from build123d import *

# Parameters (mm, degrees)
SKETCH1_R           = 3
BOSS_EXTRUDE3_DEPTH = 8
SKETCH2_R           = 4.75
CUT_EXTRUDE1_DEPTH  = 109.271164213


with BuildPart() as part:
    # Sketch1 → Boss-Extrude3 (new body)
    # profile 1 of 5: a face of its own
    with BuildSketch(Plane.XY):
        with BuildLine():
            ThreePointArc((76.35, 0), (53.987602744, 53.987602744), (0, 76.35))
            ThreePointArc((0, 76.35), (-62.014972319, 44.536116897), (-72.348554199, -24.392810524))
            ThreePointArc((-72.348554199, -24.392810524), (-44.536116897, -62.014972319), (0, -76.35))
            ThreePointArc((0, -76.35), (53.987602744, -53.987602744), (76.35, 0))
        make_face()
        Polygon((-27.25, -54.236860279), (-24.5, -59), (-27.25, -63.763139721), (-32.75, -63.763139721), (-35.5, -59), (-32.75, -54.236860279), align=None, mode=Mode.SUBTRACT)
        Polygon((54.236860279, -27.25), (59, -24.5), (63.763139721, -27.25), (63.763139721, -32.75), (59, -35.5), (54.236860279, -32.75), align=None, mode=Mode.SUBTRACT)
        Polygon((-54.236860279, 27.25), (-59, 24.5), (-63.763139721, 27.25), (-63.763139721, 32.75), (-59, 35.5), (-54.236860279, 32.75), align=None, mode=Mode.SUBTRACT)
        Polygon((27.25, 54.236860279), (24.5, 59), (27.25, 63.763139721), (32.75, 63.763139721), (35.5, 59), (32.75, 54.236860279), align=None, mode=Mode.SUBTRACT)
    # profile 2 of 5: a face of its own
    with BuildSketch(Plane.XY):
        Polygon((-63.763139721, 32.75), (-63.763139721, 27.25), (-59, 24.5), (-54.236860279, 27.25), (-54.236860279, 32.75), (-59, 35.5), align=None)
        with Locations((-59, 30)):
            Circle(SKETCH1_R, mode=Mode.SUBTRACT)
    # profile 3 of 5: a face of its own
    with BuildSketch(Plane.XY):
        Polygon((32.75, 63.763139721), (27.25, 63.763139721), (24.5, 59), (27.25, 54.236860279), (32.75, 54.236860279), (35.5, 59), align=None)
        with Locations((30, 59)):
            Circle(SKETCH1_R, mode=Mode.SUBTRACT)
    # profile 4 of 5: a face of its own
    with BuildSketch(Plane.XY):
        Polygon((63.763139721, -32.75), (63.763139721, -27.25), (59, -24.5), (54.236860279, -27.25), (54.236860279, -32.75), (59, -35.5), align=None)
        with Locations((59, -30)):
            Circle(SKETCH1_R, mode=Mode.SUBTRACT)
    # profile 5 of 5: a face of its own
    with BuildSketch(Plane.XY):
        Polygon((-32.75, -63.763139721), (-27.25, -63.763139721), (-24.5, -59), (-27.25, -54.236860279), (-32.75, -54.236860279), (-35.5, -59), align=None)
        with Locations((-30, -59)):
            Circle(SKETCH1_R, mode=Mode.SUBTRACT)
    extrude(amount=BOSS_EXTRUDE3_DEPTH)

    # Sketch2 → Cut-Extrude1 (cut, through all)
    with BuildSketch(Plane.XY.offset(8)):
        Circle(SKETCH2_R)
    extrude(amount=-CUT_EXTRUDE1_DEPTH, mode=Mode.SUBTRACT)


solid = part.part
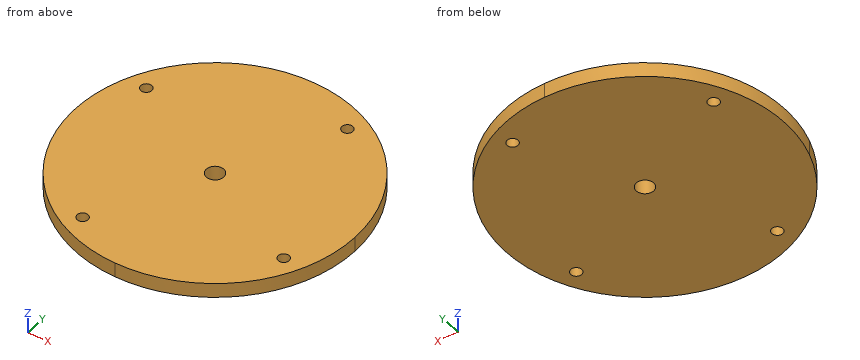
Model file for the job. Use its own axes, mm. Coordinates: 2 decimals unless noted, no trailing zeros. Write each loop counter-clockwise with the first axis right and the second up, starting at its lowest first coordinate (ties: lowest second). Pieces come first, ordered by that corner, then holes. Notation, with made-up numbers: (5.25, -31) - (32.25, -31) arc R22 cw to (32.25, 4) - close; hole circle Ø11 at (49, 33). An arc over 180 degrees is marked (long way). Write each question's results on one line, items separated by ' | '. Start each with the question number.
1) Probe line 1 along Y through (x, z) = (0, 3); line 2 along Y through (x, z) = (-59, 4.5); line 3 along X through (y, z) = (31, 2.25). List the from-to ranges inside material, lowest first. Write a range as from..to.
2) Cut at B-B (y = 30). Write the cut outline in (x, z).
3) Flat gauge pins, fed straight in: P1, Ø1, axis at y = -44, z = 1.5, coming from the -X side; P2, Ø1, axis at x = 55.5, z = 1, coming from the +Y side; P3, Ø4, axis at y = -21, z = 3, coming from the +X side; P4, Ø5, axis at x = -59, y = 30, coming from the +Z side. Where does each tip first touch, or does it go through?
4) Cut at A-A (z = 6.75). Write the cut outline in (x, y).
5) Cut at C-C (x = 59). Write the cut outline in (y, z).
6) Cut at D-D (x = -15). Write the cut outline in (y, z).
Returned:
1) line 1: -76.35..-4.75, 4.75..76.35 | line 2: -48.46..27, 33..48.46 | line 3: -69.77..-61.83, -56.17..69.77
2) outline: (-70.21, 0) - (-62, 0) - (-62, 8) - (-70.21, 8) - close; (-56, 0) - (70.21, 0) - (70.21, 8) - (-56, 8) - close
3) P1: x = -62.75 | P2: y = 52.96 | P3: x = 73.95 | P4: through
4) outline: circle Ø152.7 at (0, 0); hole circle Ø6 at (-59, 30); hole circle Ø6 at (-30, -59); hole circle Ø9.5 at (0, 0); hole circle Ø6 at (30, 59); hole circle Ø6 at (59, -30)
5) outline: (-48.46, 0) - (-33, 0) - (-33, 8) - (-48.46, 8) - close; (-27, 0) - (48.46, 0) - (48.46, 8) - (-27, 8) - close
6) outline: (-74.86, 0) - (74.86, 0) - (74.86, 8) - (-74.86, 8) - close
